Source: CAD feature listing. Evaluate the final solid. Frame: model axes, mm. Face numbers are marked on the shaded views. A direction names the side the tool comes from. Coordinates: 2 decimals unless noted, no trailing zeros. Loops run counter-clockwise (first coordinate to the right, second up) from the corner with the lowest first, then second, coordinate; pieces in that order, holes last.
Autodesk Inventor part; units mm, degrees
ref_plane "YZ Plane" through (0, 0, 0) normal (1, 0, 0) x (0, 1, 0)
ref_plane "XZ Plane" through (0, 0, 0) normal (0, 1, 0) x (-1, 0, 0)
ref_plane "XY Plane" through (0, 0, 0) normal (0, 0, 1) x (1, 0, 0)
sketch "Эскиз1" plane through (0, 0, 0) normal (0, 0, 1) x (1, 0, 0)
  arc A0 (16.937, 4.4032) -> (-11.9308, -12.8026) centre (0, 0) ccw
  arc A1 (22.4785, 0.9844) -> (-22.5, 0) centre (0, 0) ccw
  line L0 (-22.5, 0) -> (-22.5, -55)
  line L1 (-22.5, 0) -> (32.5, 0) construction
  line L2 (-22.5, -55) -> (-17.5, -55)
  line L3 (21.6965, 0.5499) -> (17.743, 3.256)
  arc A2 (-11.3173, -14.5681) -> (-11.9308, -12.8026) centre (-13.2943, -14.2658) ccw
  arc A3 (16.937, 4.4032) -> (17.743, 3.256) centre (18.8727, 4.9064) ccw
  arc A4 (21.6965, 0.5499) -> (22.4785, 0.9844) centre (21.9789, 0.9626) ccw
  line L4 (-11.3173, -14.5681) -> (-11.3173, -55)
  line L5 (-11.3173, -55) -> (-17.5, -55)
  point P0 (22.5, 0)
  point P1 (-11.1519, -13.4865)
  point P2 (17.1061, 3.6919)
  dimension "d0" = 35
  dimension "d1" = 45
  dimension "d2" = 55
  dimension "d3" = 90
  dimension "d4" = 5
  dimension "d5" = 2
  dimension "d6" = 0.5
extrude "Выдавливание1" add sketch "Эскиз1" along normal blind 25
sketch "Эскиз2" plane through (0, 0, 25) normal (0, 0, 1) x (1, 0, 0)
  line L0 (-22.5, -55) -> (-11.3173, -55)
  line L1 (-16.9086, -55) -> (-16.9086, -49)
  circle A0 centre (-16.9086, -49) radius 2
  line L2 (-16.9086, -49) -> (-16.9086, -33)
  circle A1 centre (-16.9086, -33) radius 2
  point P0 (0, 0)
  dimension "d9" = 6
  dimension "d10" = 4
  dimension "d11" = 16
  dimension "d12" = 4
extrude "Выдавливание2" cut sketch "Эскиз2" against normal blind 10
sketch "Эскиз3" plane through (-22.5, -55, 0) normal (-1, 0, 0) x (0, 0, 1)
  line L0 (25, 24) -> (25, 20)
  line L1 (25, 8) -> (25, 4)
  line L2 (25, 20) -> (25, 18.5)
  line L3 (25, 8) -> (25, 11)
  line L4 (0, 55) -> (0, 0)
  line L5 (25, 18.5) -> (0, 18.5)
  line L6 (0, 18.5) -> (0, 9.5)
  line L7 (0, 9.5) -> (25, 9.5)
  line L8 (25, 9.5) -> (25, 18.5)
  line L9 (21.8, 18.5) -> (21.8, 9.5)
  line L10 (21.8, 18.5) -> (13.8, 18.5)
  line L11 (13.8, 18.5) -> (13.8, 9.5)
  line L12 (21.8, 9.5) -> (13.8, 9.5)
  line L13 (25, 24) -> (25, 25.5)
  line L14 (21.8, 18.5) -> (13.8, 18.5)
  line L15 (25, 24) -> (25, 4)
  line L16 (25, 14) -> (-3.5354, 14)
  line L17 (21.8, 9.5) -> (13.8, 9.5)
  line L18 (25, 4) -> (25, 2.5)
  line L19 (25, 20) -> (15, 20)
  line L20 (21.8, 20) -> (13.8, 20)
  line L21 (13.8, 20) -> (13.8, 25.5)
  line L22 (13.8, 25.5) -> (21.8, 25.5)
  line L23 (21.8, 25.5) -> (21.8, 20)
  line L24 (21.8, 8) -> (13.8, 8)
  line L25 (13.8, 8) -> (13.8, 2.5)
  line L26 (13.8, 2.5) -> (21.8, 2.5)
  line L27 (21.8, 2.5) -> (21.8, 8)
  line L28 (21.8, 18.5) -> (13.8, 18.5)
  line L29 (13.8, 18.5) -> (13.8, 20)
  line L30 (13.8, 20) -> (21.8, 20)
  line L31 (21.8, 20) -> (21.8, 18.5)
  line L32 (21.8, 8) -> (13.8, 8)
  line L33 (13.8, 8) -> (13.8, 9.5)
  line L34 (13.8, 9.5) -> (21.8, 9.5)
  line L35 (21.8, 9.5) -> (21.8, 8)
  point P0 (15, 8)
  point P1 (21.8, 9.5)
  point P2 (13.8, 9.5)
  dimension "d15" = 1.5
  dimension "d16" = 3
  dimension "d18" = 8
  dimension "d21" = 1.5
extrude "Выдавливание3" cut sketch "Эскиз3" against normal through all contours L31 L5 L29 L20 L19 | L19 L20 L21 L22 L23 | L35 L24 L33 L7 | L27 L26 L25 L24
sketch "Эскиз4" plane through (-22.5, -55, 0) normal (0, -1, 0) x (1, 0, 0)
  line L0 (0, 0) -> (11.1827, 0)
  line L1 (11.1827, 0) -> (11.1827, 25)
  line L2 (0, 25) -> (11.1827, 25)
  line L3 (0, 0) -> (0, 25)
  point P0 (22.5, 0)
extrude "Выдавливание4" add sketch "Эскиз4" along normal blind 0.7
sketch "Эскиз5" plane through (-22.5, 0, 0) normal (-1, 0, 0) x (0, 0, 1)
  line L0 (13.8, -52.5) -> (21.8, -52.5)
  line L1 (0, 0) -> (0, -55.7)
  line L2 (9.8, -52.5) -> (0, 0)
  line L3 (25, -55.7) -> (0, -55.7)
  line L4 (9.8, -52.5) -> (10.3973, -55.7)
  dimension "d24" = 4
extrude "Выдавливание5" cut sketch "Эскиз5" against normal through all
fillet "Сопряжение1" radius 2 4 edges at (-16.9086, -36.5, 13.8) (-16.9086, -29.5, 13.8) (-16.9086, -52.5, 13.8) (-16.9086, -45.5, 13.8)
fillet "Сопряжение2" radius 2 1 edges at (-16.9086, -55.7, 25)
properties part number "крюк"
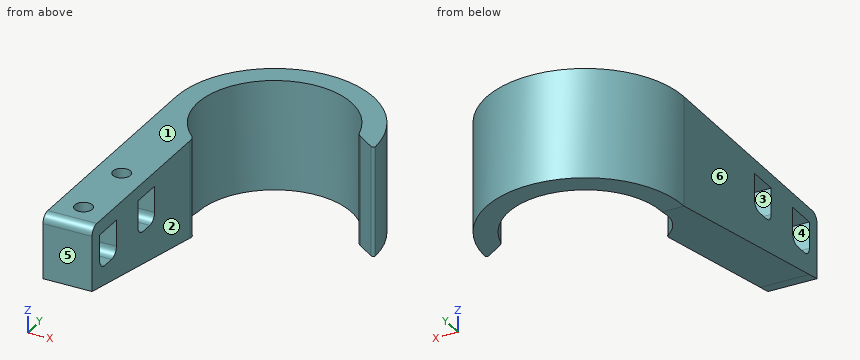
Q1. Section A-A, the plane y = -33. Return the cut outline in (x, z).
Q2. Section D-D, the plane x = -6. Return the cut outline in (y, z), plus the area to 3 significant figures.
Q3. Section C-C, the plane z = 11.25. Return the cut outline in (x, y).
Q4. Section B-B, the plane y = 10. Return the cut outline in (x, z), plus the area to 3 significant figures.
Q5. Access query for the marked faces 1 and 2. Directions: +Z, -Z, +X, -X, +Y, -Y. A direction counts if a zero-diameter tool reaches every point of the face in a straight line with its end or side. Return the directions, or none.
Q6. Line query: line 1 along X through (y, z) = (-49, 23.05); line 2 along X through (y, z) = (-19, 17); line 3 along Y through (x, z) = (-11.5, 13.25). Output: solid intervals per line, ascending.
Q7. Draft query along Y for the marked faces 3, 4, 5 and 6. Return one class per face: +Y half, -Y half, draft (parallel to the pull), parting line (faces both ways), or undercut.
Q8. Contact query for flat-ended pins moving along their axis: pin 1 Ø3.5 at (x, y) = (-16.91, -33) entering from +Z; pin 2 Ø5 at (x, z) = (-16, 20) entering from +Y; pin 3 Ø3 at (x, z) = (-16.5, 19) entering from +Y. Output: stop coordinate, or through.
Derived:
1. outline: (-22.5, 6.16) - (-11.32, 6.16) - (-11.32, 13.8) - (-22.5, 13.8) - close; (-22.5, 21.8) - (-18.91, 21.8) - (-18.91, 25) - (-22.5, 25) - close; (-14.91, 21.8) - (-11.32, 21.8) - (-11.32, 25) - (-14.91, 25) - close
2. outline: (16.44, 0) - (21.69, 0) - (21.69, 25) - (16.44, 25) - close
2. area: 131 mm2
3. outline: (-22.5, -55.7) - (-11.32, -55.7) - (-11.32, -14.57) arc R2 ccw to (-11.93, -12.8) arc R17.5 cw (long way) to (16.94, 4.4) arc R2 ccw to (17.74, 3.26) - (21.7, 0.55) arc R0.5 ccw to (22.48, 0.98) arc R22.5 ccw to (-22.5, 0) - close
4. outline: (-20.16, 0) - (-14.36, 0) - (-14.36, 25) - (-20.16, 25) - close; (14.36, 0) - (20.16, 0) - (20.16, 25) - (14.36, 25) - close
4. area: 290 mm2
5. face 1: +Z, +X, -X, +Y, -Y
5. face 2: +Z, -Z, +X, -Y
6. line 1: x = -22.5 to -18.91, -14.91 to -11.32
6. line 2: x = -22.5 to -11.32
6. line 3: y = -55.7 to -13.38, 13.19 to 19.34
7. face 3: undercut
7. face 4: undercut
7. face 5: -Y half
7. face 6: draft
8. pin 1: stops at z = 13.82
8. pin 2: stops at y = 18
8. pin 3: stops at y = 16.77
